```python
from build123d import *

# Parameters (mm, degrees)
SKETCH1_R           = 50
SKETCH1_R_2         = 2
BOSS_EXTRUDE1_DEPTH = 10
SKETCH3_R           = 21
CUT_EXTRUDE2_DEPTH  = 5
SKETCH3_4_R         = 1.75
CUT_EXTRUDE3_DEPTH  = 11
SKETCH3_5_R         = 10
CUT_EXTRUDE4_DEPTH  = 11


with BuildPart() as part:
    # Sketch1 → Boss-Extrude1 (new body)
    with BuildSketch(Plane(origin=(0, 0, 0), x_dir=(1, 0, 0), z_dir=(0, 1, 0))):
        Circle(SKETCH1_R)
        with BuildLine():
            ThreePointArc((-28.385488932, 31.921022838), (-31.921022838, 31.921022838), (-31.921022838, 28.385488932))
            Line((-31.921022838, 28.385488932), (-21.31442112, 17.778887214))
            ThreePointArc((-21.31442112, 17.778887214), (-17.778887214, 17.778887214), (-17.778887214, 21.31442112))
            Line((-17.778887214, 21.31442112), (-28.385488932, 31.921022838))
        make_face(mode=Mode.SUBTRACT)
        with BuildLine():
            ThreePointArc((-31.921022838, -28.385488932), (-31.921022838, -31.921022838), (-28.385488932, -31.921022838))
            Line((-28.385488932, -31.921022838), (-17.778887214, -21.31442112))
            ThreePointArc((-17.778887214, -21.31442112), (-17.778887214, -17.778887214), (-21.31442112, -17.778887214))
            Line((-21.31442112, -17.778887214), (-31.921022838, -28.385488932))
        make_face(mode=Mode.SUBTRACT)
        with BuildLine():
            ThreePointArc((28.385488932, -31.921022838), (31.921022838, -31.921022838), (31.921022838, -28.385488932))
            Line((31.921022838, -28.385488932), (21.31442112, -17.778887214))
            ThreePointArc((21.31442112, -17.778887214), (17.778887214, -17.778887214), (17.778887214, -21.31442112))
            Line((17.778887214, -21.31442112), (28.385488932, -31.921022838))
        make_face(mode=Mode.SUBTRACT)
        with BuildLine():
            ThreePointArc((31.921022838, 28.385488932), (31.921022838, 31.921022838), (28.385488932, 31.921022838))
            Line((28.385488932, 31.921022838), (17.778887214, 21.31442112))
            ThreePointArc((17.778887214, 21.31442112), (17.778887214, 17.778887214), (21.31442112, 17.778887214))
            Line((21.31442112, 17.778887214), (31.921022838, 28.385488932))
        make_face(mode=Mode.SUBTRACT)
        with BuildLine():
            ThreePointArc((-46.077281732, 19.413503243), (-35.355339059, 35.355339059), (-19.413503243, 46.077281732))
            ThreePointArc((-19.413503243, 46.077281732), (-25.799706685, 45.41900176), (-31.466251763, 48.436814511))
            ThreePointArc((-31.466251763, 48.436814511), (-48.436814511, 48.436814511), (-48.436814511, 31.466251763))
            ThreePointArc((-48.436814511, 31.466251763), (-45.41900176, 25.799706685), (-46.077281732, 19.413503243))
        make_face()
        with Locations((-39.951533137, 39.951533137)):
            Circle(SKETCH1_R_2, mode=Mode.SUBTRACT)
        with BuildLine():
            ThreePointArc((-31.466251763, -48.436814511), (-25.799706685, -45.41900176), (-19.413503243, -46.077281732))
            ThreePointArc((-19.413503243, -46.077281732), (-35.355339059, -35.355339059), (-46.077281732, -19.413503243))
            ThreePointArc((-46.077281732, -19.413503243), (-45.41900176, -25.799706685), (-48.436814511, -31.466251763))
            ThreePointArc((-48.436814511, -31.466251763), (-48.436814511, -48.436814511), (-31.466251763, -48.436814511))
        make_face()
        with Locations((-39.951533137, -39.951533137)):
            Circle(SKETCH1_R_2, mode=Mode.SUBTRACT)
        with BuildLine():
            ThreePointArc((48.436814511, -31.466251763), (45.41900176, -25.799706685), (46.077281732, -19.413503243))
            ThreePointArc((46.077281732, -19.413503243), (35.355339059, -35.355339059), (19.413503243, -46.077281732))
            ThreePointArc((19.413503243, -46.077281732), (25.799706685, -45.41900176), (31.466251763, -48.436814511))
            ThreePointArc((31.466251763, -48.436814511), (48.436814511, -48.436814511), (48.436814511, -31.466251763))
        make_face()
        with Locations((39.951533137, -39.951533137)):
            Circle(SKETCH1_R_2, mode=Mode.SUBTRACT)
        with BuildLine():
            ThreePointArc((19.413503243, 46.077281732), (35.355339059, 35.355339059), (46.077281732, 19.413503243))
            ThreePointArc((46.077281732, 19.413503243), (45.41900176, 25.799706685), (48.436814511, 31.466251763))
            ThreePointArc((48.436814511, 31.466251763), (48.436814511, 48.436814511), (31.466251763, 48.436814511))
            ThreePointArc((31.466251763, 48.436814511), (25.799706685, 45.41900176), (19.413503243, 46.077281732))
        make_face()
        with Locations((39.951533137, 39.951533137)):
            Circle(SKETCH1_R_2, mode=Mode.SUBTRACT)
    extrude(amount=BOSS_EXTRUDE1_DEPTH)

    # Sketch3 → Cut-Extrude2 (cut)
    with BuildSketch(Plane.XZ):
        Circle(SKETCH3_R)
    extrude(amount=-CUT_EXTRUDE2_DEPTH, mode=Mode.SUBTRACT)

    # Sketch3_4 → Cut-Extrude3 (cut, through all)
    with BuildSketch(Plane.XZ):
        with Locations((0, 14.5)):
            Circle(SKETCH3_4_R)
        with Locations((12.557368355, -7.25)):
            Circle(SKETCH3_4_R)
        with Locations((-12.557368355, -7.25)):
            Circle(SKETCH3_4_R)
    extrude(amount=-CUT_EXTRUDE3_DEPTH, mode=Mode.SUBTRACT)

    # Sketch3_5 → Cut-Extrude4 (cut, through all)
    with BuildSketch(Plane.XZ):
        Circle(SKETCH3_5_R)
    extrude(amount=-CUT_EXTRUDE4_DEPTH, mode=Mode.SUBTRACT)


solid = part.part
```
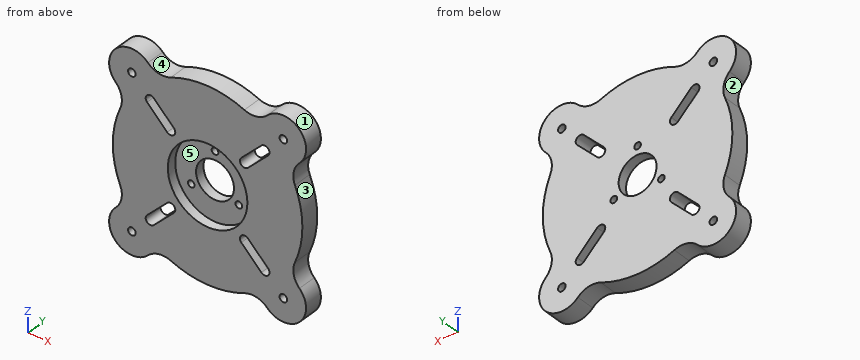
Could you check a few things on this model? Use its own coordinates, in mm. Face numbers are marked on the shaded views. A direction names the side the tool comes from. Round coordinates to 2 decimals unless told otherwise and drop trailing zeros. Loops run counter-clockwise (first coordinate to the right, second up) from the corner with the lowest first, then second, coordinate; pieces in that order, holes last. Notation, with made-up numbers: (58.25, -16) - (67.25, -16) arc R13 ccw to (67.25, -7) - close; hole circle Ø6 at (2.5, 67). An arc over 180 degrees is marked (long way). Answer in a Markdown table with one row per item. Add a question column.
(1) If we section it at C-C (z = -15): Please give me the cut outline in (x, y), plus the area to 3 significant figures.
(2) If we section it at D-D (y = 7.75): State how many separate pieces and enclosed holes the cut face has, plus the area to 3 significant figures.
(3) If we section it at A-A (z = 0): Please give me the cut outline in (x, y), plus the area to 3 significant figures.
(4) If we mould it in two halves opening along X, with no side actions, what happens to the marked faces 1, 2 and 3? For each: pulls with the +X half, pulls with the -X half, needs draft (parallel to the pull), parting line crosses it, or undercut.
(5) I'm going to push flat-ended pins straight in: pin 1 (3 mm diameter, centred on y = 4, z = -6.5, fed in from +X); pin 2 (1.5 mm diameter, centred on x = 38.5, y = 7.5, fed in from +Z); pin 3 (1.5 mm diameter, centred on y = 6.5, z = -33.5, fed in from +X). Where does each tip first touch, or does it pass through?
(6) If we section it at B-B (x = 3): Please give me the cut outline in (y, z).
(7) I need wall thicknesses on line 1 along Z through (x, y) = (-17.5, 2); line 2 along Z through (x, y) = (28, 2.75); line 3 along X through (y, z) = (9.75, 41). Which ranges of each line are inside material? Lowest first, please.
(8) For the marked faces 4 and 5, which set-ups out of +Z, -Z, +X, -X, +Y, -Y let a thin tool reach every point of the face, with its end or its side?
Model answer:
| question | item | result |
|---|---|---|
| 1 | outline | (-47.7, 0) - (-14.7, 0) - (-14.7, 5) - (14.7, 5) - (14.7, 0) - (47.7, 0) - (47.7, 10) - (-47.7, 10) - close |
| 1 | area | 807 mm² |
| 2 | separate pieces | 1 |
| 2 | enclosed holes | 12 |
| 2 | area | 8,750 mm² |
| 3 | outline | (-50, 0) - (-21, 0) - (-21, 5) - (-10, 5) - (-10, 10) - (-50, 10) - close; (10, 5) - (21, 5) - (21, 0) - (50, 0) - (50, 10) - (10, 10) - close |
| 3 | area | 690 mm² |
| 4 | face 1 | undercut |
| 4 | face 2 | pulls with the -X half |
| 4 | face 3 | pulls with the +X half |
| 5 | pin 1 | stops at x = 49.75 |
| 5 | pin 2 | stops at z = 51.93 |
| 5 | pin 3 | stops at x = 50.51 |
| 6 | outline | (0, -49.91) - (10, -49.91) - (10, -9.54) - (5, -9.54) - (5, -20.78) - (0, -20.78) - close; (0, 20.78) - (5, 20.78) - (5, 9.54) - (10, 9.54) - (10, 49.91) - (0, 49.91) - close |
| 7 | line 1 | z = -46.84 to -20.98, -18.11 to -11.61, 11.61 to 18.11, 20.98 to 46.84 |
| 7 | line 2 | z = -46.1 to -31.54, -24.46 to 24.46, 31.54 to 46.1 |
| 7 | line 3 | x = -51.91 to -41.65, -38.25 to 38.25, 41.65 to 51.91 |
| 8 | face 4 | +Z, +Y, -Y |
| 8 | face 5 | -Y |
